```python
from build123d import *

# Parameters (mm, degrees)
SKETCH1_R           = 92.5
SKETCH1_R_2         = 2
BOSS_EXTRUDE1_DEPTH = 3
BOSS_EXTRUDE2_START = 3
SKETCH1_3_R         = 35
SKETCH1_3_R_2       = 30
BOSS_EXTRUDE2_DEPTH = 5


with BuildPart() as part:
    # Sketch1 → Boss-Extrude1 (new body)
    with BuildSketch(Plane(origin=(0, 0, 0), x_dir=(1, 0, 0), z_dir=(0, 1, 0))):
        with Locations(Location((0, 0, 0), (0, 0, 270))):
            Circle(SKETCH1_R)
        with Locations(Location((-81.663945533, 30, 0), (0, 0, 270))):
            Circle(SKETCH1_R_2, mode=Mode.SUBTRACT)
        with Locations(Location((81.663945533, 30, 0), (0, 0, 270))):
            Circle(SKETCH1_R_2, mode=Mode.SUBTRACT)
        with Locations(Location((13.609798459, 85.928885632, 0), (0, 0, 270))):
            Circle(SKETCH1_R_2, mode=Mode.SUBTRACT)
        with Locations(Location((13.609798459, -85.928885632, 0), (0, 0, 270))):
            Circle(SKETCH1_R_2, mode=Mode.SUBTRACT)
        with Locations(Location((-13.609798459, 85.928885632, 0), (0, 0, 270))):
            Circle(SKETCH1_R_2, mode=Mode.SUBTRACT)
        with Locations(Location((-13.609798459, -85.928885632, 0), (0, 0, 270))):
            Circle(SKETCH1_R_2, mode=Mode.SUBTRACT)
        with Locations(Location((81.663945533, -30, 0), (0, 0, 270))):
            Circle(SKETCH1_R_2, mode=Mode.SUBTRACT)
        with Locations(Location((-81.663945533, -30, 0), (0, 0, 270))):
            Circle(SKETCH1_R_2, mode=Mode.SUBTRACT)
    extrude(amount=BOSS_EXTRUDE1_DEPTH)

    # Sketch1_3 → Boss-Extrude2 (add)
    with BuildSketch(Plane(origin=(0, 0, 0), x_dir=(1, 0, 0), z_dir=(0, 1, 0)).offset(BOSS_EXTRUDE2_START)):
        with Locations(Location((0, 0, 0), (0, 0, 270))):
            Circle(SKETCH1_3_R)
        with Locations(Location((0, 0, 0), (0, 0, 270))):
            Circle(SKETCH1_3_R_2, mode=Mode.SUBTRACT)
    extrude(amount=BOSS_EXTRUDE2_DEPTH)

    # Sketch2 → Cut-Revolve1 (revolve, cut)
    with BuildSketch(Plane.XY, mode=Mode.PRIVATE) as cut_revolve1_sk:
        with BuildLine():
            Line((35, 6), (35, 4))
            ThreePointArc((35, 4), (34, 5), (35, 6))
        make_face()
    revolve(cut_revolve1_sk.sketch.rotate(Axis((0, 0, 0), (0, 1, 0)), 90), axis=Axis((0, 0, 0), (0, 1, 0)), mode=Mode.SUBTRACT)


solid = part.part
```
Could you check a few things on this model? Use its own coordinates, in mm. A direction names the side the tool comes from. Give positions to 0.01 mm unless a question says otherwise; leave off trailing zeros. Loops run counter-clockwise (first coordinate to the right, second up) from the corner with the lowest first, then second, coordinate; pieces in that order, holes last. Notation, with made-up numbers: (44.5, -10.5) -> (51.5, -10.5) arc R18 cw to (51.5, 1.5) -> close; hole circle Ø6 at (66.25, -10.75). An arc over 180 degrees is marked (long way). Put each result on its own line as item: value.
(1) Please list where these lines run through material, in increasing order: probe 1 along Y at (x, z) = (-8, -83); probe 2 along X at (y, z) = (7, 27.5); probe 3 along X at (y, z) = (1.6, 30). Write a range as [from, to].
Computed:
probe 1: [0, 3]
probe 2: [-21.65, -11.99], [11.99, 21.65]
probe 3: [-87.5, -83.66], [-79.66, 79.66], [83.66, 87.5]
(2) Imagine slicing it at B-B on z = 0. Write out the boundary of the cut face in (x, y), plus the area to 3 significant figures.
Computed:
outline: (-92.5, 0) -> (92.5, 0) -> (92.5, 3) -> (35, 3) -> (35, 4) arc R1 cw to (35, 6) -> (35, 8) -> (30, 8) -> (30, 3) -> (-30, 3) -> (-30, 8) -> (-35, 8) -> (-35, 6) arc R1 cw to (-35, 4) -> (-35, 3) -> (-92.5, 3) -> close
area: 602 mm^2
(3) Imagine slicing it at A-A on x = 0. Write out the boundary of the cut face in (y, z), plus the area to 3 significant figures.
Computed:
outline: (0, -92.5) -> (3, -92.5) -> (3, -35) -> (4, -35) arc R1 cw to (6, -35) -> (8, -35) -> (8, -30) -> (3, -30) -> (3, 30) -> (8, 30) -> (8, 35) -> (6, 35) arc R1 cw to (4, 35) -> (3, 35) -> (3, 92.5) -> (0, 92.5) -> close
area: 602 mm^2
(4) Imagine slicing it at C-C on y = 1.25. State how many separate pieces and enclosed holes the cut face has, plus the area to 3 significant figures.
Computed:
separate pieces: 1
enclosed holes: 8
area: 26,800 mm^2
(5) I'm going to push flat-ended pins straight in: pin 1 Ø3 at (x, y) = (30.5, 6.5) entering from -Z; pin 2 Ø2 at (y, z) = (6.5, -4) entering from +X; pin 3 Ø2.5 at (x, z) = (-81.66, -30) entering from -Y; pin 4 Ø6.5 at (x, z) = (-13.61, 85.93) entering from +Y. Where does each tip first touch, or does it pass through?
Computed:
pin 1: z = -19.6
pin 2: x = 34.87
pin 3: through
pin 4: y = 3
(6) Imagine slicing it at D-D on x = 52. Write out the boundary of the cut face in (y, z).
Computed:
outline: (0, -76.5) -> (3, -76.5) -> (3, 76.5) -> (0, 76.5) -> close
(7) Thinking about a two-plate mould opening in X: for faces 3 (the face through (-21.3, 3.49, -27.77)), 4 (the face through (-83.616, 1.479, 29.566)), 5 (the face through (1, 3, 40)), which applies, pulls with the +X half, pulls with the -X half, needs draft (parallel to the pull), parting line crosses it, or undercut?
Computed:
face 3: parting line crosses it
face 4: undercut
face 5: needs draft
(8) For faces 1 (the face through (-13.01, 1.48, -84.02)), 2 (the face through (0, 3, 0)), which set-ups out of +Z, -Z, +X, -X, +Y, -Y let a thin tool reach every point of the face, with its end or its side?
Computed:
face 1: +Y, -Y
face 2: +Y
